For this review, take the finished solid that the model builds, in its own axes (mm). Round coordinates to 2 decimals unless told otherwise and drop trailing zeros. Loops run counter-clockwise (first coordinate to the right, second up) from the corner with the lowest first, then second, coordinate; pieces in that order, holes last. Notation, with made-up numbers: M -31.5,46.25 L -10.5,46.25 A19 ccw -10.5,60.25 Z; hole C 30.5,78.5 d2. An arc over 180 degrees is marked long. One line per question, with ' | ' between items. Start each with the question number.
1) For pin 1 Ø1 at (x, y) = (-22.5, 11) entering from +Z; pin 2 Ø3 at (x, y) = (-98.5, 3.5) entering from -Z; pin 3 Ø1.5 at (x, y) = (-60.5, 10) entering from -Z; pin 4 Ø12 at (x, z) = (-100, 68.5) entering from -Y, all flat-tipped, find the tip position at first contact; note any pin that passes through.
2) For probe 1 along X at (y, z) = (8.5, 39); probe 2 along X at (y, z) = (8.5, 90); probe 3 along Z at (x, y) = (-17, 7), list the stretches that pass through material, from the lowest coordinate up. Write a range as from..to.
3) We need section A-A (y = 4.5). Give the boundary of the cut face in (x, z).
```python
from build123d import *

# Parameters (mm, degrees)
F1_R = 12.7


with BuildPart() as f2:
    # F2: sweep along a path in F0
    with BuildLine(Plane.XZ) as f2_path:
        ThreePointArc((139.7, 0), (0, 139.7), (-139.7, 0))
    # F1 (on Top) → F2 (sweep)
    with BuildSketch(Plane.XY):
        with Locations((-139.7, 0)):
            Circle(F1_R)
    sweep(path=f2_path.line)

    # F4: sweep along a path in F0
    with BuildLine(Plane.XZ) as f4_path:
        ThreePointArc((139.7, 0), (0, 139.7), (-139.7, 0))
    # F3 (on face) → F4 (sweep, cut)
    with BuildSketch(Plane(origin=(0, 0, 0), x_dir=(1, 0, 0), z_dir=(0, 0, -1))):
        with BuildLine():
            ThreePointArc((-152.4, 0), (-139.7, 12.3904935703), (-127, 0))
            ThreePointArc((-127, 0), (-139.7, 12.7), (-152.4, 0))
        make_face()
        with BuildLine():
            Line((-152.4, 0), (-127, 0))
            ThreePointArc((-127, 0), (-139.7, 12.3904935703), (-152.4, 0))
        make_face()
    sweep(path=f4_path.line, mode=Mode.SUBTRACT)

    # F6: sweep along a path in F0
    with BuildLine(Plane.XZ) as f6_path:
        ThreePointArc((139.7, 0), (0, 139.7), (-139.7, 0))
    # F5 (on face) → F6 (sweep, cut)
    with BuildSketch(Plane(origin=(0, 0, 0), x_dir=(1, 0, 0), z_dir=(0, 0, -1))):
        with BuildLine():
            ThreePointArc((-128.5875, 0), (-139.7, 11.1125), (-150.8125, 0))
            Line((-150.8125, 0), (-128.5875, 0))
        make_face()
        with BuildLine():
            Line((-128.5875, 0), (-150.8125, 0))
            ThreePointArc((-150.8125, 0), (-139.7, -11.1125), (-128.5875, 0))
        make_face()
    sweep(path=f6_path.line, mode=Mode.SUBTRACT)


solid = f2.part
```
Answers below:
1) pin 1: z = 145.11 | pin 2: z = 78.98 | pin 3: z = 116.11 | pin 4: y = 0
2) probe 1: -143.95..-141.58, -126.67..-124.29, 124.29..126.67, 141.58..143.95 | probe 2: -118.92..-116.05, -97.3..-94.17, 94.17..97.3, 116.05..118.92 | probe 3: 127.98..129.96, 147.35..149.33
3) outline: M -151.58,0 L -149.86,0 A149.86 cw 149.86,0 L 151.58,0 A151.58 ccw Z; M -129.54,0 L -127.82,0 A127.82 cw 127.82,0 L 129.54,0 A129.54 ccw Z
